from build123d import *

# Parameters (mm, degrees)
SKETCH1_W           = 25.4
SKETCH1_H           = 25.4
SKETCH1_W_2         = 19.05
SKETCH1_H_2         = 19.05
BOSS_EXTRUDE1_DEPTH = 254
SKETCH2_R           = 2.0193
CUT_EXTRUDE1_DEPTH  = 635
SKETCH3_R           = 2.0193
CUT_EXTRUDE2_DEPTH  = 635


with BuildPart() as part:
    # Sketch1 → Boss-Extrude1 (new body)
    with BuildSketch(Plane(origin=(0, 0, 0), x_dir=(1, 0, 0), z_dir=(0, 1, 0))):
        with Locations((12.7, 12.7)):
            Rectangle(SKETCH1_W, SKETCH1_H)
        with Locations((12.7, 12.7)):
            Rectangle(SKETCH1_W_2, SKETCH1_H_2, mode=Mode.SUBTRACT)
    extrude(amount=BOSS_EXTRUDE1_DEPTH)

    # Sketch2 → Cut-Extrude1 (cut)
    with BuildSketch(Plane.XY):
        with Locations((12.7, 12.7)):
            Circle(SKETCH2_R)
        with Locations((12.7, 25.4)):
            Circle(SKETCH2_R)
        with Locations((12.7, 38.1)):
            Circle(SKETCH2_R)
        with Locations((12.7, 50.8)):
            Circle(SKETCH2_R)
        with Locations((12.7, 63.5)):
            Circle(SKETCH2_R)
        with Locations((12.7, 76.2)):
            Circle(SKETCH2_R)
        with Locations((12.7, 88.9)):
            Circle(SKETCH2_R)
        with Locations((12.7, 101.6)):
            Circle(SKETCH2_R)
        with Locations((12.7, 114.3)):
            Circle(SKETCH2_R)
        with Locations((12.7, 127)):
            Circle(SKETCH2_R)
        with Locations((12.7, 139.7)):
            Circle(SKETCH2_R)
        with Locations((12.7, 152.4)):
            Circle(SKETCH2_R)
        with Locations((12.7, 165.1)):
            Circle(SKETCH2_R)
        with Locations((12.7, 177.8)):
            Circle(SKETCH2_R)
        with Locations((12.7, 190.5)):
            Circle(SKETCH2_R)
        with Locations((12.7, 203.2)):
            Circle(SKETCH2_R)
        with Locations((12.7, 215.9)):
            Circle(SKETCH2_R)
        with Locations((12.7, 228.6)):
            Circle(SKETCH2_R)
        with Locations((12.7, 241.3)):
            Circle(SKETCH2_R)
        with Locations((12.7, 254)):
            Circle(SKETCH2_R)
        with Locations((12.7, 266.7)):
            Circle(SKETCH2_R)
        with Locations((12.7, 279.4)):
            Circle(SKETCH2_R)
        with Locations((12.7, 292.1)):
            Circle(SKETCH2_R)
        with Locations((12.7, 304.8)):
            Circle(SKETCH2_R)
        with Locations((12.7, 317.5)):
            Circle(SKETCH2_R)
        with Locations((12.7, 330.2)):
            Circle(SKETCH2_R)
        with Locations((12.7, 342.9)):
            Circle(SKETCH2_R)
        with Locations((12.7, 355.6)):
            Circle(SKETCH2_R)
        with Locations((12.7, 368.3)):
            Circle(SKETCH2_R)
        with Locations((12.7, 381)):
            Circle(SKETCH2_R)
        with Locations((12.7, 393.7)):
            Circle(SKETCH2_R)
        with Locations((12.7, 406.4)):
            Circle(SKETCH2_R)
        with Locations((12.7, 419.1)):
            Circle(SKETCH2_R)
        with Locations((12.7, 431.8)):
            Circle(SKETCH2_R)
        with Locations((12.7, 444.5)):
            Circle(SKETCH2_R)
        with Locations((12.7, 457.2)):
            Circle(SKETCH2_R)
        with Locations((12.7, 469.9)):
            Circle(SKETCH2_R)
        with Locations((12.7, 482.6)):
            Circle(SKETCH2_R)
        with Locations((12.7, 495.3)):
            Circle(SKETCH2_R)
        with Locations((12.7, 508)):
            Circle(SKETCH2_R)
        with Locations((12.7, 520.7)):
            Circle(SKETCH2_R)
        with Locations((12.7, 533.4)):
            Circle(SKETCH2_R)
        with Locations((12.7, 546.1)):
            Circle(SKETCH2_R)
        with Locations((12.7, 558.8)):
            Circle(SKETCH2_R)
        with Locations((12.7, 571.5)):
            Circle(SKETCH2_R)
        with Locations((12.7, 584.2)):
            Circle(SKETCH2_R)
        with Locations((12.7, 596.9)):
            Circle(SKETCH2_R)
        with Locations((12.7, 609.6)):
            Circle(SKETCH2_R)
        with Locations((12.7, 622.3)):
            Circle(SKETCH2_R)
    extrude(amount=-CUT_EXTRUDE1_DEPTH, mode=Mode.SUBTRACT)

    # Sketch3 → Cut-Extrude2 (cut)
    with BuildSketch(Plane(origin=(25.4, 0, 0), x_dir=(0, 0, -1), z_dir=(1, 0, 0))):
        with Locations((12.7, 12.7)):
            Circle(SKETCH3_R)
        with Locations((12.7, 25.4)):
            Circle(SKETCH3_R)
        with Locations((12.7, 38.1)):
            Circle(SKETCH3_R)
        with Locations((12.7, 50.8)):
            Circle(SKETCH3_R)
        with Locations((12.7, 63.5)):
            Circle(SKETCH3_R)
        with Locations((12.7, 76.2)):
            Circle(SKETCH3_R)
        with Locations((12.7, 88.9)):
            Circle(SKETCH3_R)
        with Locations((12.7, 101.6)):
            Circle(SKETCH3_R)
        with Locations((12.7, 114.3)):
            Circle(SKETCH3_R)
        with Locations((12.7, 127)):
            Circle(SKETCH3_R)
        with Locations((12.7, 139.7)):
            Circle(SKETCH3_R)
        with Locations((12.7, 152.4)):
            Circle(SKETCH3_R)
        with Locations((12.7, 165.1)):
            Circle(SKETCH3_R)
        with Locations((12.7, 177.8)):
            Circle(SKETCH3_R)
        with Locations((12.7, 190.5)):
            Circle(SKETCH3_R)
        with Locations((12.7, 203.2)):
            Circle(SKETCH3_R)
        with Locations((12.7, 215.9)):
            Circle(SKETCH3_R)
        with Locations((12.7, 228.6)):
            Circle(SKETCH3_R)
        with Locations((12.7, 241.3)):
            Circle(SKETCH3_R)
        with Locations((12.7, 254)):
            Circle(SKETCH3_R)
        with Locations((12.7, 266.7)):
            Circle(SKETCH3_R)
        with Locations((12.7, 279.4)):
            Circle(SKETCH3_R)
        with Locations((12.7, 292.1)):
            Circle(SKETCH3_R)
        with Locations((12.7, 304.8)):
            Circle(SKETCH3_R)
        with Locations((12.7, 317.5)):
            Circle(SKETCH3_R)
        with Locations((12.7, 330.2)):
            Circle(SKETCH3_R)
        with Locations((12.7, 342.9)):
            Circle(SKETCH3_R)
        with Locations((12.7, 355.6)):
            Circle(SKETCH3_R)
        with Locations((12.7, 368.3)):
            Circle(SKETCH3_R)
        with Locations((12.7, 381)):
            Circle(SKETCH3_R)
        with Locations((12.7, 393.7)):
            Circle(SKETCH3_R)
        with Locations((12.7, 406.4)):
            Circle(SKETCH3_R)
        with Locations((12.7, 419.1)):
            Circle(SKETCH3_R)
        with Locations((12.7, 431.8)):
            Circle(SKETCH3_R)
        with Locations((12.7, 444.5)):
            Circle(SKETCH3_R)
        with Locations((12.7, 457.2)):
            Circle(SKETCH3_R)
        with Locations((12.7, 469.9)):
            Circle(SKETCH3_R)
        with Locations((12.7, 482.6)):
            Circle(SKETCH3_R)
        with Locations((12.7, 495.3)):
            Circle(SKETCH3_R)
        with Locations((12.7, 508)):
            Circle(SKETCH3_R)
        with Locations((12.7, 520.7)):
            Circle(SKETCH3_R)
        with Locations((12.7, 533.4)):
            Circle(SKETCH3_R)
        with Locations((12.7, 546.1)):
            Circle(SKETCH3_R)
        with Locations((12.7, 558.8)):
            Circle(SKETCH3_R)
        with Locations((12.7, 571.5)):
            Circle(SKETCH3_R)
        with Locations((12.7, 584.2)):
            Circle(SKETCH3_R)
        with Locations((12.7, 596.9)):
            Circle(SKETCH3_R)
        with Locations((12.7, 609.6)):
            Circle(SKETCH3_R)
        with Locations((12.7, 622.3)):
            Circle(SKETCH3_R)
    extrude(amount=-CUT_EXTRUDE2_DEPTH, mode=Mode.SUBTRACT)


solid = part.part
Source: CAD feature listing. Evaluate the final solid. Frame: model axes, mm. A direction names the side the tool comes from. Coordinates: 2 decimals unless noted, no trailing zeros. Write each loop counter-clockwise with the first axis right and the second up, starting at its lowest first coordinate (ties: lowest second). Pieces come first, ordered by that corner, then holes. Notation, with made-up numbers: M -9,72.25 L 22,72.25 A22 cw 22,81.25 Z; hole C 68,28.25 d8. An arc over 180 degrees is marked long. Use a Markdown table: item, result.
1) Section B-B, the plane x = 7. Output: boundary loops of the cut face in (y, z) (3 decimals), then the cut area to 3 significant figures.
Conclusion:
| item | result |
|---|---|
| outline | M 0,-25.4 L 254,-25.4 L 254,-22.225 L 0,-22.225 Z; M 0,-3.175 L 254,-3.175 L 254,0 L 0,0 Z |
| area | 1,610 mm^2 |
2) Reachability of faces 1 (the flat face through (10, 125, -3.175)), 2 (the cylindrical face through (12.437, 90.902, -1.565)) from +Z, -Z, +X, -X, +Y, -Y: full face, straight path, thin tool, end or side. Return the list, or none.
Conclusion:
| item | result |
|---|---|
| face 1 | +Y, -Y |
| face 2 | +Z, -Z |
3) First-contact query: pin 1 Ø6.5 at (x, y) = (12.7, 88.9) entering from -Z. Flat tip, straight axial feed; report the tip coordinate or a pass-through.
Conclusion:
| item | result |
|---|---|
| pin 1 | stops at z = -25.4 |
4) Section A-A, the plane z = -7.75. Output: boundary loops of the cut face in (x, y) (3 decimals).
Conclusion:
| item | result |
|---|---|
| outline | M 0,0 L 3.175,0 L 3.175,254 L 0,254 Z; M 22.225,0 L 25.4,0 L 25.4,254 L 22.225,254 Z |
5) Ray query, L1, parallel to X at y = 193.5, z = -12 (3 decimals); L2, parallel to Z at x = 21, y = 184.5 (3 decimals); L3, parallel to X at y = 228.6, z = -1.7. Return the intervals inside material, ascending.
Conclusion:
| item | result |
|---|---|
| L1 | x = 0 to 3.175, 22.225 to 25.4 |
| L2 | z = -25.4 to -22.225, -3.175 to 0 |
| L3 | x = 0 to 10.68, 14.72 to 25.4 |
6) Mould query, pull axis Z, two halves, no side actions, for faces 3 (the cylindrical face through (12.26, 201.23, -23.79)), 4 (the cylindrical face through (1.61, 90.902, -12.437)), 5 (the flat face through (15, 125, -25.4)). Classes: pulls with the +Z half, pulls with the -Z half, needs draft (parallel to the pull), parting line crosses it, or undercut.
Conclusion:
| item | result |
|---|---|
| face 3 | needs draft |
| face 4 | undercut |
| face 5 | pulls with the -Z half |
